Source: CAD feature listing. Evaluate the final solid. Frame: model axes, mm. Coordinates: 2 decimals unless noted, no trailing zeros. Order: outer loops, then holes, each group sorted by start corner. A loop starts at its lowest first (then second) coordinate and runs counter-clockwise, first axis right, second up. Notation, with made-up numbers: (-14.5, 57.25) -> (-3.5, 57.25) arc R18 cw to (-3.5, 85.25) -> close; hole circle Ø5 at (23.5, 88.5). An arc over 180 degrees is marked (long way). Put each result on its own line as item: value.
from build123d import *

# Parameters (mm, degrees)
F1_DEPTH = 19.05


with BuildPart() as f1:
    # F0 (on Front) → F1 (new body)
    with BuildSketch(Plane.XZ):
        with BuildLine():
            Line((-114.3, 457.2), (-202.373318, -297.714158))
            ThreePointArc((-202.373318, -297.714158), (-200.809256, -302.67196), (-196.066097, -304.8))
            Line((-196.066097, -304.8), (-106.763423, -304.8))
            ThreePointArc((-106.763423, -304.8), (-102.757269, -303.376786), (-100.546898, -299.74511))
            Line((-100.546898, -299.74511), (-42.312409, -20.219562))
            ThreePointArc((-42.312409, -20.219562), (-33.470926, -5.692855), (-17.446306, 0))
            Line((-17.446306, 0), (17.446306, 0))
            ThreePointArc((17.446306, 0), (33.470926, -5.692855), (42.312409, -20.219562))
            Line((42.312409, -20.219562), (100.546898, -299.74511))
            ThreePointArc((100.546898, -299.74511), (102.757269, -303.376786), (106.763423, -304.8))
            Line((106.763423, -304.8), (196.066097, -304.8))
            ThreePointArc((196.066097, -304.8), (200.809256, -302.67196), (202.373318, -297.714158))
            Line((202.373318, -297.714158), (114.3, 457.2))
            Line((114.3, 457.2), (9.525, 457.2))
            Line((9.525, 457.2), (9.525, 235.204))
            ThreePointArc((9.525, 235.204), (12.827, 231.902), (9.525, 228.6))
            Line((9.525, 228.6), (-9.525, 228.6))
            ThreePointArc((-9.525, 228.6), (-12.827, 231.902), (-9.525, 235.204))
            Line((-9.525, 235.204), (-9.525, 457.2))
            Line((-9.525, 457.2), (-114.3, 457.2))
        make_face()
    extrude(amount=F1_DEPTH)


solid = f1.part
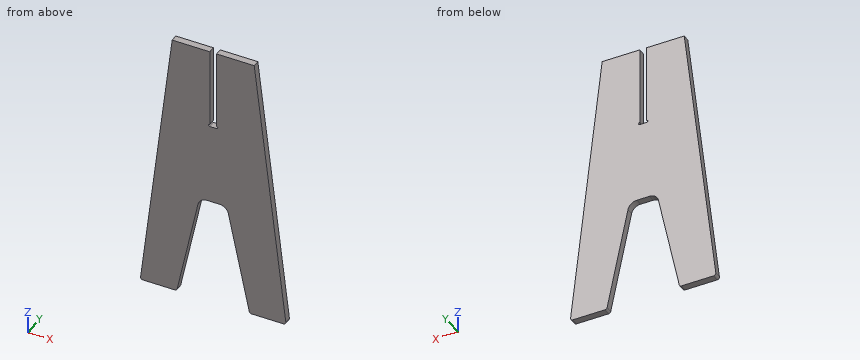
1. Ray query, line 1 along X through (y, z) = (-2.5, 349) (3 decimals); line 2 along X through (y, z) = (-7.25, -263); line 3 along X through (y, z) = (-6.5, 227). Return the intervals inside material, ascending.
Numbers:
line 1: x = -126.923 to -9.525, 9.525 to 126.923
line 2: x = -198.32 to -92.89, 92.89 to 198.32
line 3: x = -141.16 to 141.16
2. Cut plane A-A on z = -225.5. Output: boundary loops of the cut face in (x, y), plus the area to 3 significant figures.
Numbers:
outline: (-193.95, -19.05) -> (-85.08, -19.05) -> (-85.08, 0) -> (-193.95, 0) -> close; (85.08, -19.05) -> (193.95, -19.05) -> (193.95, 0) -> (85.08, 0) -> close
area: 4,150 mm2
3. Cut plane B-B on y = -12. Output: boundary loops of the cut face in (x, z) (3 decimals), plus the area to 3 significant figures.
Numbers:
outline: (-202.373, -297.714) arc R6.35 ccw to (-196.066, -304.8) -> (-106.763, -304.8) arc R6.35 ccw to (-100.547, -299.745) -> (-42.312, -20.22) arc R25.4 cw to (-17.446, 0) -> (17.446, 0) arc R25.4 cw to (42.312, -20.22) -> (100.547, -299.745) arc R6.35 ccw to (106.763, -304.8) -> (196.066, -304.8) arc R6.35 ccw to (202.373, -297.714) -> (114.3, 457.2) -> (9.525, 457.2) -> (9.525, 235.204) arc R3.302 cw to (9.525, 228.6) -> (-9.525, 228.6) arc R3.302 cw to (-9.525, 235.204) -> (-9.525, 457.2) -> (-114.3, 457.2) -> close
area: 195,000 mm2
4. Cut plane C-C on z = -143. Output: boundary loops of the cut face in (x, y), plus the area to 3 significant figures.
Numbers:
outline: (-184.32, -19.05) -> (-67.89, -19.05) -> (-67.89, 0) -> (-184.32, 0) -> close; (67.89, -19.05) -> (184.32, -19.05) -> (184.32, 0) -> (67.89, 0) -> close
area: 4,440 mm2
5. Cut plane D-D on x = 162.5. Output: boundary loops of the cut face in (y, z), plus the area to 3 significant figures.
Numbers:
outline: (-19.05, -304.8) -> (0, -304.8) -> (0, 44.06) -> (-19.05, 44.06) -> close
area: 6,650 mm2
6. First-contact query: pin 1 (6 mm diameter, centred on y = -7.5, z = 267.5, fed in from -X); pin 2 (6 mm diameter, centred on y = -5.5, z = -89.5, fed in from -X); pin 3 (5.5 mm diameter, centred on x = -2.5, y = -8.5, fed in from -Z). Flat tips, straight axial feed; report the tip coordinate or a pass-through.
Numbers:
pin 1: stops at x = -136.78
pin 2: stops at x = -178.43
pin 3: stops at z = 0
